The listing builds one solid part. Answer for the finished solid, in the listing's coordinates (mm). A direction names the side the tool comes from. Coordinates: 2 decimals unless noted, no trailing zeros. Order: outer loops, then holes, each group sorted by start corner. A loop starts at its lowest first (then second) coordinate and runs counter-clockwise, first axis right, second up. Notation, with made-up numbers: (-12, 5) -> (17, 5) arc R30 ccw to (17, 44) -> close; hole circle Ø9 at (68.25, 29). An arc over 180 degrees is marked (long way). Return JSON: item names as keys, results as strings.
from build123d import *

# Parameters (mm, degrees)
SKETCH1_W               = 28
SKETCH1_H               = 30
BOSS_EXTRUDE1_DEPTH     = 32.5
CUT_EXTRUDE1_DEPTH      = 53.347397261
CUT_EXTRUDE1_DEPTH_BACK = 53.347397261
SKETCH2_W               = 20
SKETCH2_H               = 21
CUT_EXTRUDE2_DEPTH      = 53.347397261
CUT_EXTRUDE2_DEPTH_BACK = 53.347397261
SKETCH3_W               = 12
SKETCH3_H               = 8.5
CUT_EXTRUDE3_DEPTH      = 53.347397261
CUT_EXTRUDE3_DEPTH_BACK = 53.347397261


with BuildPart() as part:
    # Sketch1 → Boss-Extrude1 (new body)
    with BuildSketch(Plane(origin=(0, 0, 0), x_dir=(1, 0, 0), z_dir=(0, 1, 0))):
        with Locations((14, 15)):
            Rectangle(SKETCH1_W, SKETCH1_H)
    extrude(amount=BOSS_EXTRUDE1_DEPTH)

    # Sketch2 → Cut-Extrude1 (cut, two sides: drawn at the far end of the back side and taken through both)
    with BuildSketch(Plane.XY.offset(-CUT_EXTRUDE1_DEPTH_BACK)):
        with Locations((14, 12)):
            Rectangle(SKETCH2_W, SKETCH2_H)
    extrude(amount=CUT_EXTRUDE1_DEPTH + CUT_EXTRUDE1_DEPTH_BACK, mode=Mode.SUBTRACT)

    # Sketch3 → Cut-Extrude2 (cut, two sides: drawn at the far end of the back side and taken through both)
    with BuildSketch(Plane.XY.offset(-CUT_EXTRUDE2_DEPTH_BACK)):
        with Locations((14, 26.75)):
            Rectangle(SKETCH3_W, SKETCH3_H)
    extrude(amount=CUT_EXTRUDE2_DEPTH + CUT_EXTRUDE2_DEPTH_BACK, mode=Mode.SUBTRACT)

    # Sketch4 → Cut-Extrude3 (cut, two sides: drawn at the far end of the back side and taken through both)
    with BuildSketch(Plane.XY.offset(-CUT_EXTRUDE3_DEPTH_BACK)):
        Polygon((8, 22.5), (8, 23.5), (7.5, 22.5), align=None)
        Polygon((4, 22.5), (3.5, 22.5), (4, 21.5), align=None)
        Polygon((20, 22.5), (20, 23.5), (20.5, 22.5), align=None)
        Polygon((8, 31), (7.5, 31), (8, 30), align=None)
        Polygon((20, 31), (20.5, 31), (20, 30), align=None)
        Polygon((24, 22.5), (24.5, 22.5), (24, 21.5), align=None)
        Polygon((24, 1.5), (24.5, 1.5), (24, 2.5), align=None)
        Polygon((4, 1.5), (3.5, 1.5), (4, 2.5), align=None)
    extrude(amount=CUT_EXTRUDE3_DEPTH + CUT_EXTRUDE3_DEPTH_BACK, mode=Mode.SUBTRACT)


solid = part.part
1. Consider line 1 (Y direction, x = 18, z = -11); line 2 (X direction, y = 17, z = -14.5); line 3 (Y direction, x = 6.25, z = -17). Determine where each line is inside the solid, lowest interval first. Write a range as from..to.
Answer block:
{"line 1": "y = 0..1.5, 31..32.5", "line 2": "x = 0..4, 24..28", "line 3": "y = 0..1.5, 22.5..32.5"}
2. The part is cut by section C-C on z = -19. Give the vertices of the cut face in (x, y), and give its area (3 significant figures).
Answer block:
{"outline": "(0, 0) -> (28, 0) -> (28, 32.5) -> (0, 32.5) -> close; hole (3.5, 1.5) -> (24.5, 1.5) -> (24, 2.5) -> (24, 21.5) -> (24.5, 22.5) -> (20.5, 22.5) -> (20, 23.5) -> (20, 30) -> (20.5, 31) -> (7.5, 31) -> (8, 30) -> (8, 23.5) -> (7.5, 22.5) -> (3.5, 22.5) -> (4, 21.5) -> (4, 2.5) -> close", "area": "386 mm2"}
3. The part is cut by section A-A on x = 22. Give the vertices of the cut face in (y, z).
Answer block:
{"outline": "(0, -30) -> (1.5, -30) -> (1.5, 0) -> (0, 0) -> close; (22.5, -30) -> (32.5, -30) -> (32.5, 0) -> (22.5, 0) -> close"}
4. Determine the mould class of faces 1 (the face through (0, 16, -15)), 2 (the face through (14, 32.5, -15)), 3 (the face through (7.754, 23.007, -15.21)) for opening direction X: pulls with the +X half, pulls with the -X half, needs draft (parallel to the pull), parting line crosses it, or undercut.
Answer block:
{"face 1": "pulls with the -X half", "face 2": "needs draft", "face 3": "undercut"}
5. For faces 4 (the face through (14, 1.5, -15)), 5 (the face through (28, 16, -15)), determine the directions among +Z, -Z, +X, -X, +Y, -Y from which every point of the face is accessible in a straight line to the end or side of a thin tool.
Answer block:
{"face 4": "+Z, -Z", "face 5": "+Z, -Z, +X, +Y, -Y"}
6. The part is cut by section B-B on y = 23. Give the vertices of the cut face in (x, z).
Answer block:
{"outline": "(0, -30) -> (7.75, -30) -> (7.75, 0) -> (0, 0) -> close; (20.25, -30) -> (28, -30) -> (28, 0) -> (20.25, 0) -> close"}
